Could you check a few things on this model? Use its own coordinates, in mm. Face numbers are marked on the shaded views. A direction names the side the tool comes from. Give positions to 0.01 mm unless a question says otherwise; leave off trailing zeros. Write each loop counter-clockwise with the first axis right and the second up, starting at its lowest first coordinate (ties: lowest second). Pieces come first, ordered by that corner, then holes. Notation, with made-up numbers: (19, 31.25) - (42, 31.25) arc R21 cw to (42, 45.25) - close; hole circle Ø10 at (40.5, 82.5). An arc over 180 degrees is marked (long way). Answer in a Markdown table with one row per item.
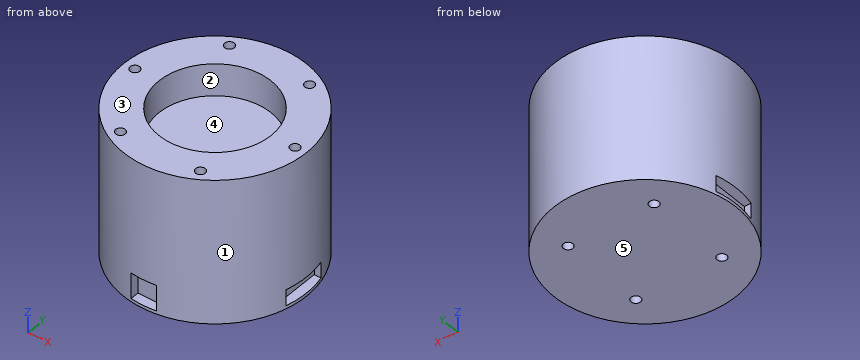
from build123d import *

# Parameters (mm, degrees)
SKETCH_1_R               = 28.5
EXTRUDE_1_DEPTH          = 45
SKETCH_2_R               = 1.5
CUT_EXTRUDE_1_DEPTH      = 5
PATTERN_CIRCULAR_1_COUNT = 6
SKETCH_3_R               = 17.5
CUT_EXTRUDE_2_DEPTH      = 10
CUT_EXTRUDE_START        = -1
CUT_EXTRUDE_3_DEPTH      = 5
CUT_EXTRUDE_4_DEPTH      = 8
SKETCH_6_R               = 1.5
CUT_EXTRUDE_5_DEPTH      = 4
PATTERN_CIRCULAR_2_COUNT = 4


with BuildPart() as part:
    # 草图1 → 凸台-拉伸1 (new body)
    with BuildSketch(Plane.XY):
        with Locations(Location((0, 0, 0), (0, 0, 180))):
            Circle(SKETCH_1_R)
    extrude(amount=EXTRUDE_1_DEPTH)

    # 草图2 → 切除-拉伸1 (cut)
    with BuildSketch(Plane.XY.offset(45)):
        with Locations((25, 0)):
            Circle(SKETCH_2_R)
    cut_extrude_1 = extrude(amount=-CUT_EXTRUDE_1_DEPTH, mode=Mode.SUBTRACT)

    # 阵列(圆周)1: 切除-拉伸1 ×6 about axis
    pattern_circular_1_axis = Axis((0, 0, 0), (0, 0, 1))
    for i in range(1, PATTERN_CIRCULAR_1_COUNT):
        add(cut_extrude_1.rotate(pattern_circular_1_axis, i * 360 / PATTERN_CIRCULAR_1_COUNT), mode=Mode.SUBTRACT)

    # 草图3 → 切除-拉伸2 (cut)
    with BuildSketch(Plane.XY.offset(45)):
        Circle(SKETCH_3_R)
    extrude(amount=-CUT_EXTRUDE_2_DEPTH, mode=Mode.SUBTRACT)

    # 草图4 → 切除-拉伸3 (cut)
    with BuildSketch(Plane(origin=(0, 0, 0), x_dir=(-1, 0, 0), z_dir=(0, 0, -1)).offset(CUT_EXTRUDE_START)):
        with BuildLine():
            Line((-25.5, -7), (-27.689719766, -7))
            ThreePointArc((-27.689719766, -7), (-28.56082248, 0), (-27.689719766, 7))
            Line((-27.689719766, 7), (-25.5, 7))
            Line((-25.5, 7), (-25.5, -7))
        make_face()
        with BuildLine():
            Line((25.5, 7), (27.689719766, 7))
            ThreePointArc((27.689719766, 7), (28.56082248, 0), (27.689719766, -7))
            Line((27.689719766, -7), (25.5, -7))
            Line((25.5, -7), (25.5, 7))
        make_face()
    extrude(amount=-CUT_EXTRUDE_3_DEPTH, mode=Mode.SUBTRACT)

    # 草图5 → 切除-拉伸4 (cut)
    with BuildSketch(Plane(origin=(0, 0, 0), x_dir=(-1, 0, 0), z_dir=(0, 0, -1)).offset(CUT_EXTRUDE_START)):
        with BuildLine():
            Line((-4, -25.5), (4, -25.5))
            Line((4, -25.5), (4, -28.217902119))
            ThreePointArc((4, -28.217902119), (0, -28.5), (-4, -28.217902119))
            Line((-4, -28.217902119), (-4, -25.5))
        make_face()
    extrude(amount=-CUT_EXTRUDE_4_DEPTH, mode=Mode.SUBTRACT)

    # 草图6 → 切除-拉伸5 (cut)
    with BuildSketch(Plane(origin=(0, 0, 0), x_dir=(-1, 0, 0), z_dir=(0, 0, -1))):
        with Locations((13.435028843, 13.435028843)):
            Circle(SKETCH_6_R)
    cut_extrude_5 = extrude(amount=-CUT_EXTRUDE_5_DEPTH, mode=Mode.SUBTRACT)

    # 阵列(圆周)2: 切除-拉伸5 ×4 about axis
    pattern_circular_2_axis = Axis((0, 0, 0), (0, 0, 1))
    for i in range(1, PATTERN_CIRCULAR_2_COUNT):
        add(cut_extrude_5.rotate(pattern_circular_2_axis, i * 360 / PATTERN_CIRCULAR_2_COUNT), mode=Mode.SUBTRACT)


solid = part.part
1) Imagine slicing it at A-A (x = 0). List the corners of the cut face in (y, z) for me.
Check values:
| item | result |
|---|---|
| outline | (-28.5, 0) - (28.5, 0) - (28.5, 45) - (17.5, 45) - (17.5, 35) - (-17.5, 35) - (-17.5, 45) - (-28.5, 45) - (-28.5, 9) - (-25.5, 9) - (-25.5, 1) - (-28.5, 1) - close |
2) Imagine slicing it at B-B (y = -5). List the corners of the cut face in (x, z) for me, then the cut area to 3 significant figures.
Check values:
| item | result |
|---|---|
| outline | (-28.06, 0) - (28.06, 0) - (28.06, 1) - (25.5, 1) - (25.5, 6) - (28.06, 6) - (28.06, 45) - (16.77, 45) - (16.77, 35) - (-16.77, 35) - (-16.77, 45) - (-28.06, 45) - (-28.06, 6) - (-25.5, 6) - (-25.5, 1) - (-28.06, 1) - close |
| area | 2,160 mm2 |
3) Will these pins go through, and if not, where does the flat tip stop? P1, Ø3, axis at y = -27, z = 6.5, coming from the -X side; P2, Ø4, axis at x = 4.5, z = 19.5, coming from the -Y side; P3, Ø1, axis at y = -14.5, z = 14, coming from the +X side.
Check values:
| item | result |
|---|---|
| P1 | stops at x = -12.73 |
| P2 | stops at y = -28.39 |
| P3 | stops at x = 24.82 |
4) On a 3-axis mill with a long thin cutter (end or side, diameter ignored), from which of +Z, -Z, +X, -X, +Y, -Y can I reach the whole of each face in a straight line? I mean the marked faces 4 and 5. Say none if no direction works.
Check values:
| item | result |
|---|---|
| face 4 | +Z |
| face 5 | -Z, +X, -X, +Y, -Y |
5) Imagine slicing it at D-D (z = 37.5). List the corners of the cut face in (x, y) for me.
Check values:
| item | result |
|---|---|
| outline | circle Ø57 at (0, 0); hole circle Ø35 at (0, 0) |
6) Imagine slicing it at C-C (z = 31). List the corners of the cut face in (x, y) for me, then the cut area to 3 significant figures.
Check values:
| item | result |
|---|---|
| outline | circle Ø57 at (0, 0) |
| area | 2,550 mm2 |
7) We'd pull the mould along X, two halves only. Please class the marked faces 1, 2 and 3: +X half, -X half, draft (parallel to the pull), parting line (faces both ways), or undercut.
Check values:
| item | result |
|---|---|
| face 1 | parting line |
| face 2 | undercut |
| face 3 | draft |
8) If I drill on line 1 (X direction, y = 7, z = 34.5); line 2 (X direction, y = 22.5, z = 25); line 3 (Z direction, x = 0, y = 3.5), over which ranges is the centre line in solid material (lowest first)?
Check values:
| item | result |
|---|---|
| line 1 | x = -27.63 to 27.63 |
| line 2 | x = -17.49 to 17.49 |
| line 3 | z = 0 to 35 |
